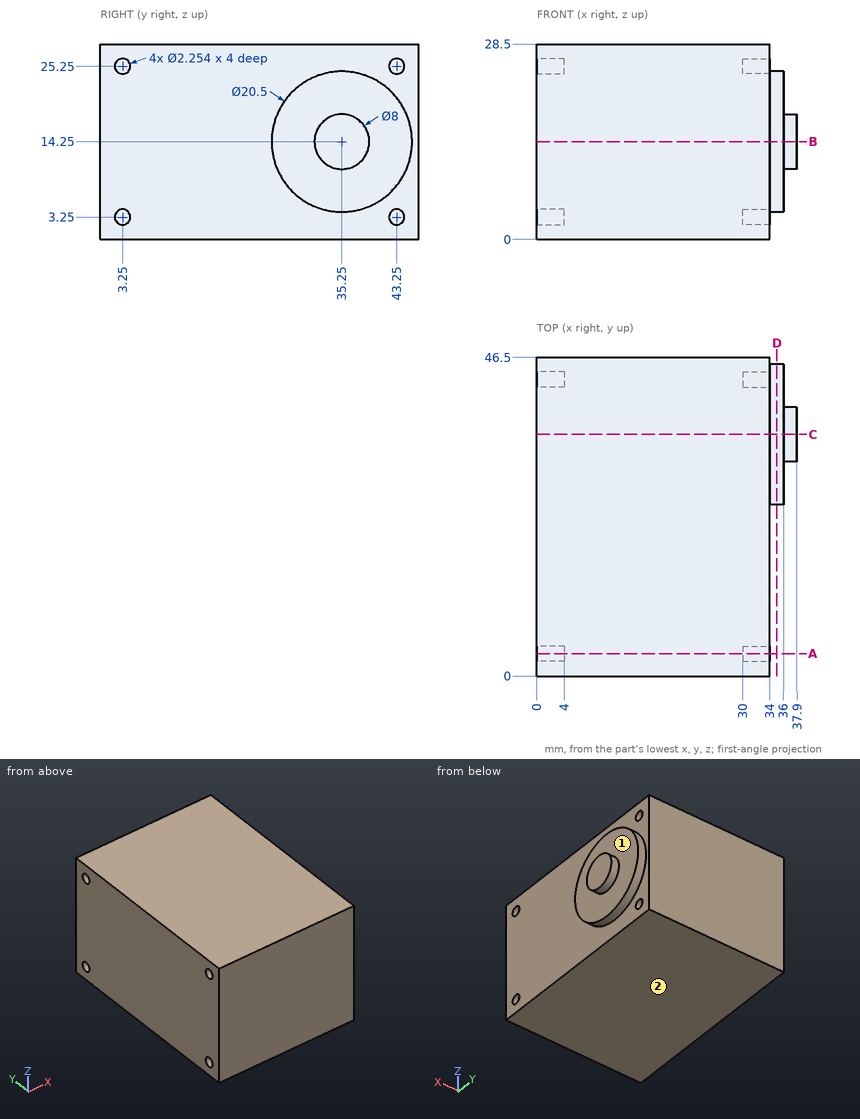
Here's the drawing with two shaded views (mm, measured from the low corner). I have some questions. A direction names the side the tool comes from. Round coordinates to 2 decimals unless told otherwise and drop trailing zeros. Write each loop counter-clockwise with the first axis right and the second up, starting at its lowest first coordinate (ties: lowest second). Pieces come first, ordered by that corner, then holes. Notation, with made-up numbers: M 74.5,15 L 123.5,15 A16 ccw 123.5,41 Z; hole C 66.5,43 d11. An arc over 180 degrees is marked long. Use CSV: the item, a comma, the result in double quotes.
(1) I need wall thicknesses on line 1 along Y through (x, z) = (31.55, 25.25); line 2 along Z through (x, y) = (31.45, 43.25); line 3 along X through (y, z) = (21, 14.75). Which ranges of each line are inside material? Lowest first, please.
Check values:
line 1,"0 to 2.12, 4.38 to 42.12, 44.38 to 46.5"
line 2,"0 to 2.12, 4.38 to 24.12, 26.38 to 28.5"
line 3,"0 to 34"
(2) Imagine slicing it at B-B (z = 14.25). Write out the boundary of the cut face in (x, y).
Check values:
outline,"M 0,0 L 34,0 L 34,25 L 36,25 L 36,31.25 L 37.9,31.25 L 37.9,39.25 L 36,39.25 L 36,45.5 L 34,45.5 L 34,46.5 L 0,46.5 Z"
(3) Imagine slicing it at A-A (y = 3.25). Write out the boundary of the cut face in (x, z), plus the area to 3 significant figures.
Check values:
outline,"M 0,0 L 34,0 L 34,2.12 L 30,2.12 L 30,4.38 L 34,4.38 L 34,24.12 L 30,24.12 L 30,26.38 L 34,26.38 L 34,28.5 L 0,28.5 L 0,26.38 L 4,26.38 L 4,24.12 L 0,24.12 L 0,4.38 L 4,4.38 L 4,2.12 L 0,2.12 Z"
area,"933 mm^2"
(4) Imagine slicing it at D-D (x = 35). Write out the boundary of the cut face in (y, z).
Check values:
outline,"C 35.25,14.25 d20.5"
(5) I'm going to push flat-ended pins straight in: pin 1 (10 mm diameter, centred on x = 6.5, y = 32, fed in from -Z); pin 2 (2.5 mm diameter, centred on y = 3, z = 25, fed in from +X); pin 3 (1.8 mm diameter, centred on y = 43.25, z = 25.25, fed in from -X); pin 4 (1.8 mm diameter, centred on y = 43.25, z = 3.25, fed in from +X). Where does each tip first touch, or does it pass through?
Check values:
pin 1,"z = 0"
pin 2,"x = 34"
pin 3,"x = 4"
pin 4,"x = 30"
(6) On a 3-axis mill with a long thin cutter (end or side, diameter ignored), from which of +Z, -Z, +X, -X, +Y, -Y can I reach the whole of each face in a straight line? I mean the marked faces 1 and 2. Say none if no direction works.
Check values:
face 1,"+X"
face 2,"-Z, +X, -X, +Y, -Y"
(7) Imagine slicing it at C-C (y = 35.25). Write out the boundary of the cut face in (x, z).
Check values:
outline,"M 0,0 L 34,0 L 34,4 L 36,4 L 36,10.25 L 37.9,10.25 L 37.9,18.25 L 36,18.25 L 36,24.5 L 34,24.5 L 34,28.5 L 0,28.5 Z"
